Print and shaded views of the part. All mm, measured from the part's lowest x, y and z. A direction names the side the tool comes from. Round coordinates to 2 decimals unless told otherwise and drop trailing zeros. Write each loop counter-clockwise with the first axis right and the second up, starting at its lowest first coordinate (ties: lowest second). Pieces come first, ordered by that corner, then holes.
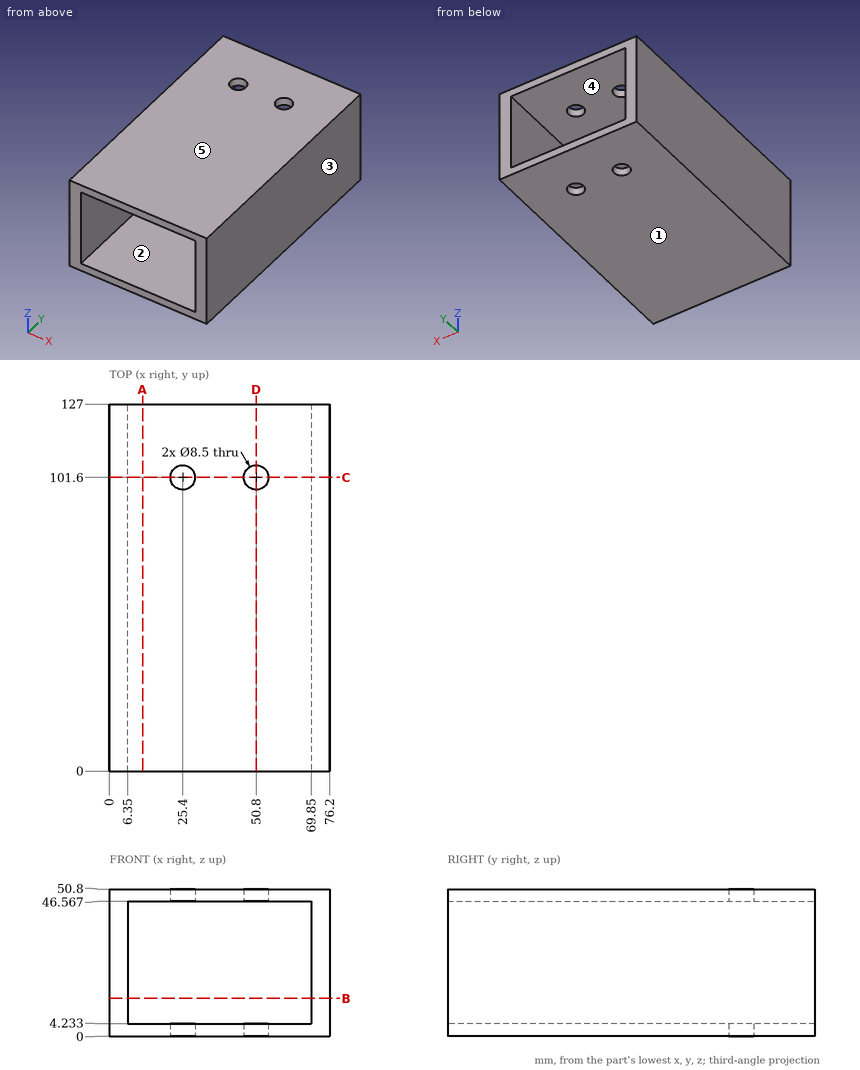
1) Slice it at D-D (x = 50.8). Write the cut outline in (y, z).
Results:
outline: (0, 0) - (97.35, 0) - (97.35, 4.23) - (0, 4.23) - close; (0, 46.57) - (97.35, 46.57) - (97.35, 50.8) - (0, 50.8) - close; (105.85, 0) - (127, 0) - (127, 4.23) - (105.85, 4.23) - close; (105.85, 46.57) - (127, 46.57) - (127, 50.8) - (105.85, 50.8) - close
2) Wall check: L1, parallel to X at y = 87, z = 31; L2, parallel to Z at x = 65.5, y = 40.5; L3, parallel to X at y = 101, z = 49. Give the ranges that are in metal, low to high.
Results:
L1: x = 0 to 6.35, 69.85 to 76.2
L2: z = 0 to 4.23, 46.57 to 50.8
L3: x = 0 to 21.19, 29.61 to 46.59, 55.01 to 76.2
3) Slice it at C-C (y = 101.6). Write the cut outline in (x, z).
Results:
outline: (0, 0) - (21.15, 0) - (21.15, 4.23) - (6.35, 4.23) - (6.35, 46.57) - (21.15, 46.57) - (21.15, 50.8) - (0, 50.8) - close; (29.65, 0) - (46.55, 0) - (46.55, 4.23) - (29.65, 4.23) - close; (29.65, 46.57) - (46.55, 46.57) - (46.55, 50.8) - (29.65, 50.8) - close; (55.05, 0) - (76.2, 0) - (76.2, 50.8) - (55.05, 50.8) - (55.05, 46.57) - (69.85, 46.57) - (69.85, 4.23) - (55.05, 4.23) - close
4) Slice it at B-B (z = 13). Write the cut outline in (x, y), plus the area to 3 significant figures.
Results:
outline: (0, 0) - (6.35, 0) - (6.35, 127) - (0, 127) - close; (69.85, 0) - (76.2, 0) - (76.2, 127) - (69.85, 127) - close
area: 1,610 mm2
5) Which spindle directions (+Z, -Z, +X, -X, +Y, -Y) get a long thin tool onto all of the face, cutting with end or side? Do the marked faces 4 and 5. Say none if no direction does.
Results:
face 4: +Y, -Y
face 5: +Z, +X, -X, +Y, -Y
6) Mould opens along X. For the marked faces 1, 2 and 3 say: released by +X, released by -X, zero draft, split by the parting line, or undercut.
Results:
face 1: zero draft
face 2: undercut
face 3: released by +X
7) Slice it at A-A (x = 11.5). Write the cut outline in (y, z).
Results:
outline: (0, 0) - (127, 0) - (127, 4.23) - (0, 4.23) - close; (0, 46.57) - (127, 46.57) - (127, 50.8) - (0, 50.8) - close
